```python
from build123d import *

# Parameters (mm, degrees)
SKETCH1_R           = 1.2
BOSS_EXTRUDE1_DEPTH = 1.5
SKETCH2_W           = 8
SKETCH2_H           = 1.5
BOSS_EXTRUDE2_DEPTH = 4
BOSS_EXTRUDE3_DEPTH = 8


with BuildPart() as part:
    # Sketch1 → Boss-Extrude1 (new body)
    with BuildSketch(Plane(origin=(0, 0, 0), x_dir=(1, 0, 0), z_dir=(0, 1, 0))):
        Polygon((-8.5, 0), (-8.5, -4), (8.5, -4), (8.5, 0), (12.5, 0), (12.5, -10), (-12.5, -10), (-12.5, 0), align=None)
        with Locations(Location((-10.5, -1.5, 0), (0, 0, 270))):
            Circle(SKETCH1_R, mode=Mode.SUBTRACT)
        with Locations(Location((10.5, -1.5, 0), (0, 0, 270))):
            Circle(SKETCH1_R, mode=Mode.SUBTRACT)
    extrude(amount=BOSS_EXTRUDE1_DEPTH)

    # Sketch2 → Boss-Extrude2 (add)
    with BuildSketch(Plane.XZ):
        with Locations((0, 9.25)):
            Rectangle(SKETCH2_W, SKETCH2_H)
    extrude(amount=BOSS_EXTRUDE2_DEPTH)

    # Sketch3 → Boss-Extrude3 (add)
    with BuildSketch(Plane.ZY.offset(4)):
        Polygon((10, -4), (4.226497308, -14), (2.726497308, -14), (8.5, -4), align=None)
    extrude(amount=-BOSS_EXTRUDE3_DEPTH)


solid = part.part
```
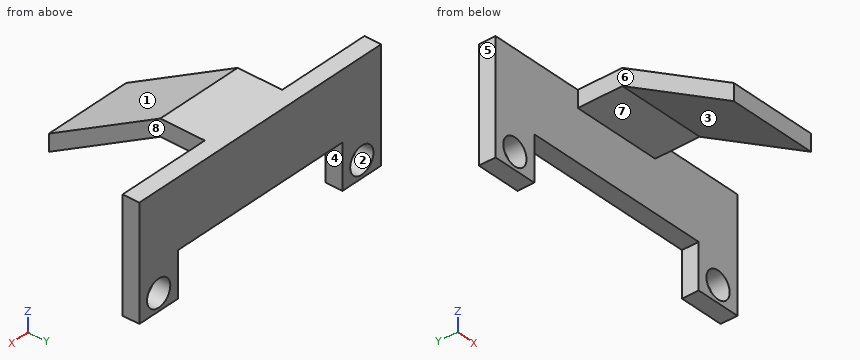
Can you work these out from the model? Positions are in its coordinate system, mm. Face numbers are marked on the shaded views. A direction names the side the tool comes from. Give positions to 0.01 mm unless a question says otherwise; leave off trailing zeros. Loops run counter-clockwise (first coordinate to the right, second up) from the corner with the lowest first, then second, coordinate; pieces in that order, holes last. Notation, with made-up numbers: M 73,-21.5 L 112,-21.5 A5 cw 112,-15.5 Z; hole C 17.5,17.5 d9. An arc over 180 degrees is marked long. One line per item, written item: value.
(1) Will these pins go through, and if not, where does the flat tip stop? pin 1 (1.2 mm diameter, centred on x = -2, y = -1.5, fed in from -Z); pin 2 (1.6 mm diameter, centred on x = -3, y = 1, fed in from -Z); pin 3 (1.5 mm diameter, centred on y = -3, z = 9, fed in from -X).
Returned:
pin 1: z = 8.5
pin 2: z = 4
pin 3: x = -4
(2) Suppose I cut it at A-A on x = -10.5. List the corners of the cut face in (y, z) for me, plus the area to 3 significant figures.
Returned:
outline: M 0,0 L 1.5,0 L 1.5,0.3 L 0,0.3 Z; M 0,2.7 L 1.5,2.7 L 1.5,10 L 0,10 Z
area: 11.4 mm^2
(3) Which directions (+Z, -Z, +X, -X, +Y, -Y) give clear straight access to the entire face, cutting with the end or side of a thin tool? Please do the marked faces 4, 5, 6, 7 and 8.
Returned:
face 4: -Z, +Y, -Y
face 5: +Z, -Z, -X, +Y, -Y
face 6: +Z, -Z, -X, -Y
face 7: -Z, +X, -X
face 8: +Z, -Z, +X, -Y
(4) I need wall thicknesses on line 1 (X direction, y = 0.5, z = 1.5); line 2 (X direction, y = -5.5, z = 7.75); line 3 (Y direction, x = -0.75, z = 6.5). Which ranges of each line are inside material? Lowest first, please.
Returned:
line 1: -12.5 to -11.7, -9.3 to -8.5, 8.5 to 9.3, 11.7 to 12.5
line 2: -4 to 4
line 3: -10.06 to -7.46, 0 to 1.5
(5) Suppose I cut it at C-C on z = 5.75. List the corners of the cut face in (x, y) for me, plus the area to 3 significant figures.
Returned:
outline: M -12.5,0 L 12.5,0 L 12.5,1.5 L -12.5,1.5 Z; M -4,-11.36 L 4,-11.36 L 4,-8.76 L -4,-8.76 Z
area: 58.3 mm^2
(6) Suppose I cut it at D-D on z = 3. List the corners of the cut face in (x, y) for me, plus the area to 3 significant figures.
Returned:
outline: M -12.5,0 L -8.5,0 L -8.5,1.5 L -12.5,1.5 Z; M -4,-14 L 4,-14 L 4,-13.53 L -4,-13.53 Z; M 8.5,0 L 12.5,0 L 12.5,1.5 L 8.5,1.5 Z
area: 15.8 mm^2
(7) Suppose I cut it at B-B on z = 1.5. List the corners of the cut face in (x, y) for me, plus the area to 3 significant figures.
Returned:
outline: M -12.5,0 L -11.7,0 L -11.7,1.5 L -12.5,1.5 Z; M -9.3,0 L -8.5,0 L -8.5,1.5 L -9.3,1.5 Z; M 8.5,0 L 9.3,0 L 9.3,1.5 L 8.5,1.5 Z; M 11.7,0 L 12.5,0 L 12.5,1.5 L 11.7,1.5 Z
area: 4.80 mm^2
(8) We'd pull the mould along Y, two halves only. Please class the marked faces 1, 2 and 3: released by +Y, released by -Y, zero draft, split by the parting line, or undercut.
Returned:
face 1: released by -Y
face 2: zero draft
face 3: undercut
